Part print with two shaded views. Sizes in mm from the minimum x, y, z corner. Coordinates: 2 decimals unless noted, no trailing zeros. Order: outer loops, then holes, each group sorted by start corner. A loop starts at its lowest first (then second) coordinate and runs counter-clockwise, first axis right, second up.
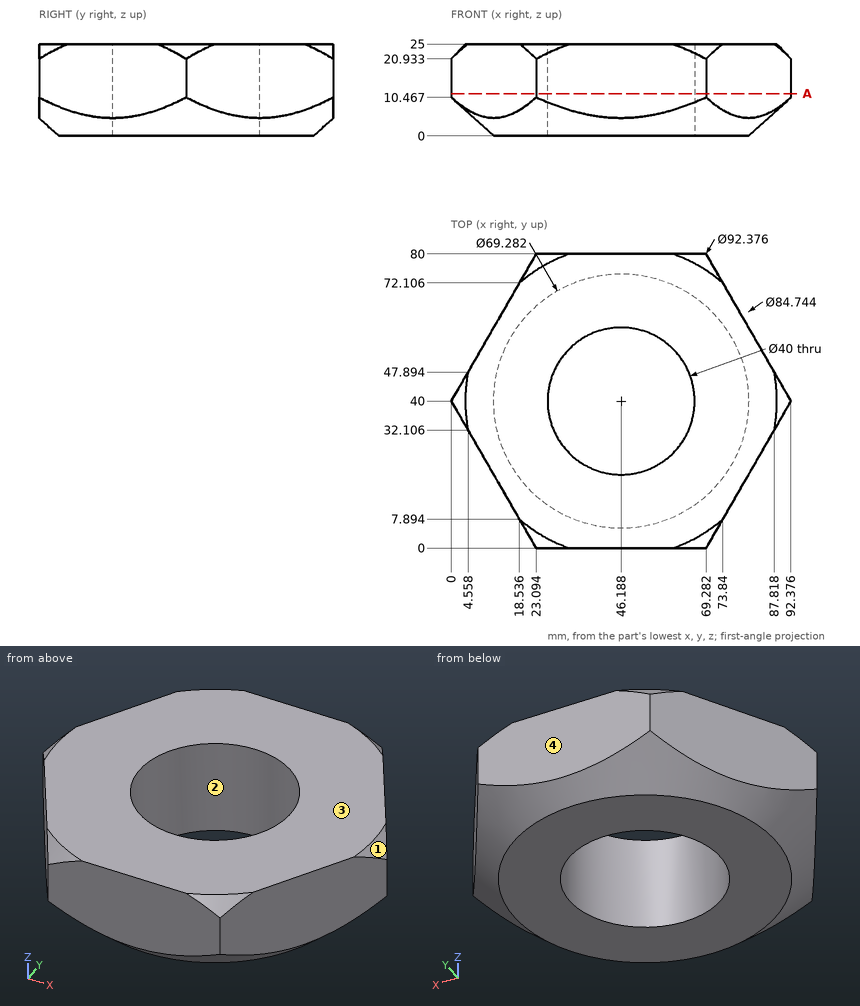
Q1. Pin check, flat tips, straight feed: pin 1 Ø1 at (x, z) = (13.5, 20) entering from -Y; pin 2 Ø3 at (x, z) = (21.5, 5.5) entering from +Y (1 decimal); pin 3 Ø3 at (x, z) = (16, 8) entering from +Y. Stop position of each tip, or through.
Results list:
pin 1: stops at y = 15.75
pin 2: stops at y = 74.7
pin 3: stops at y = 70.31
Q2. Cut at A-A on z = 11.5. Write the cut outline in (x, y), and give its area (3 significant figures).
Results list:
outline: (0, 40) - (23.09, 0) - (69.28, 0) - (92.38, 40) - (69.28, 80) - (23.09, 80) - close; hole circle Ø40 at (46.19, 40)
area: 4,290 mm2
Q3. Wall check: line 1 along Y through (x, z) = (45.5, 22); line 2 along Y through (x, z) = (61.5, 20) (1 decimal); line 3 along Y through (x, z) = (9, 21.25) (1 decimal). Give the ranges that are in metal, low to high.
Results list:
line 1: y = 0 to 20.01, 59.99 to 80
line 2: y = 0 to 27.1, 52.9 to 80
line 3: y = 24.4 to 55.6
Q4. Mould opens along Y. For the marked faces 1, 2, 3 and 4 say: pulls with the +Y half, pulls with the -Y half, needs draft (parallel to the pull), parting line crosses it, or undercut.
Results list:
face 1: parting line crosses it
face 2: undercut
face 3: needs draft
face 4: pulls with the +Y half
